The model under review builds one solid part; all positions refer to its coordinate system, in mm. A direction names the side the tool comes from. Coordinates: 2 decimals unless noted, no trailing zeros. Order: outer loops, then holes, each group sorted by start corner. A loop starts at its lowest first (then second) coordinate and runs counter-clockwise, first axis right, second up. Notation, with made-up numbers: M -33,4 L -6,4 A30 ccw -6,31 Z; hole C 45,22.5 d7. An arc over 180 degrees is marked long. Write each question's results on one line, items separated by ' | '.
from build123d import *

# Parameters (mm, degrees)
BOSS_EXTRUDE1_DEPTH     = 24
SKETCH2_W               = 3
SKETCH2_H               = 4
CUT_EXTRUDE1_DEPTH      = 4.1
BOSS_EXTRUDE2_DEPTH     = 0.8
SKETCH5_W               = 0.5
SKETCH5_H               = 0.5
CUT_EXTRUDE2_DEPTH      = 2
CUT_EXTRUDE2_DEPTH_BACK = 2
SKETCH6_W               = 1.8
SKETCH6_H               = 1.2
CUT_EXTRUDE3_DEPTH      = 0.1
SKETCH7_W               = 3
SKETCH7_H               = 1.3


with BuildPart() as part:
    # Sketch1 → Boss-Extrude1 (new body)
    with BuildSketch(Plane(origin=(0, 0, 0), x_dir=(0, 0, -1), z_dir=(1, 0, 0))):
        with BuildLine():
            Line((-2.7, 0.6), (-1.428285686, 0.6))
            ThreePointArc((-1.428285686, 0.6), (2, 2), (-1.428285686, 3.4))
            Line((-1.428285686, 3.4), (-2.7, 3.4))
            Line((-2.7, 3.4), (-2.7, 0.6))
        make_face()
    extrude(amount=BOSS_EXTRUDE1_DEPTH)

    # Sketch2 → Cut-Extrude1 (cut)
    with BuildSketch(Plane(origin=(0, 0, 0), x_dir=(0, 0, -1), z_dir=(1, 0, 0))):
        with Locations((-1.2, 2)):
            Rectangle(SKETCH2_W, SKETCH2_H)
    extrude(amount=CUT_EXTRUDE1_DEPTH, mode=Mode.SUBTRACT)

    # Sketch3 → Boss-Extrude2 (add)
    with BuildSketch(Plane.XY.offset(-0.3)):
        with BuildLine():
            Line((0.4, 0.1), (3.6, 0.1))
            ThreePointArc((3.6, 0.1), (3.812132034, 0.187867966), (3.9, 0.4))
            Line((3.9, 0.4), (3.9, 3.6))
            ThreePointArc((3.9, 3.6), (3.812132034, 3.812132034), (3.6, 3.9))
            Line((3.6, 3.9), (0.4, 3.9))
            ThreePointArc((0.4, 3.9), (0.187867966, 3.812132034), (0.1, 3.6))
            Line((0.1, 3.6), (0.1, 0.4))
            ThreePointArc((0.1, 0.4), (0.187867966, 0.187867966), (0.4, 0.1))
        make_face()
    extrude(amount=BOSS_EXTRUDE2_DEPTH)

    # Sketch4 → Revolve1 (revolve)
    with BuildSketch(Plane(origin=(0, 2, 0), x_dir=(-1, 0, 0), z_dir=(0, 1, 0))):
        Polygon((-2, 2.55), (-0.5, 2.55), (-0.5, 2.05), (0, 1.55), (0, 0.65), (-1.25, 0.65), (-1.25, 0.3), (-2, 0.3), align=None)
    revolve(axis=Axis((2, 2, 0.3), (0, 0, 1)))

    # Sketch5 → Cut-Extrude2 (cut, two sides)
    with BuildSketch(Plane(origin=(0, 2, 0), x_dir=(-1, 0, 0), z_dir=(0, 1, 0))) as cut_extrude2_sk:
        with Locations((-2, 2.3)):
            Rectangle(SKETCH5_W, SKETCH5_H)
    extrude(amount=CUT_EXTRUDE2_DEPTH, mode=Mode.SUBTRACT)
    extrude(cut_extrude2_sk.sketch, amount=-CUT_EXTRUDE2_DEPTH_BACK, mode=Mode.SUBTRACT)

    # Sketch6 → Cut-Extrude3 (cut)
    with BuildSketch(Plane.XY.offset(2.7)):
        with Locations((14.9, 2)):
            Rectangle(SKETCH6_W, SKETCH6_H)
    extrude(amount=-CUT_EXTRUDE3_DEPTH, mode=Mode.SUBTRACT)

    # Sketch7 → Revolve2 (revolve)
    with BuildSketch(Plane(origin=(0, 2, 0), x_dir=(-1, 0, 0), z_dir=(0, 1, 0))):
        with Locations((-25.5, -0.65)):
            Rectangle(SKETCH7_W, SKETCH7_H)
    revolve(axis=Axis((27, 2, 0), (-1, 0, 0)))


solid = part.part
1) For faces 4 (the flat face through (1, 2, 0.65)), 5 (the flat face through (4.1, 2, 2)), 6 (the cylindrical face through (0.5, 2, 2.3)), 7 (the flat face through (3, 2, 2.55)), 8 (the flat face through (15, 2, 2.6)), list the 3-axis set-ups (+Z, -Z, +X, -X, +Y, -Y) from which the entire face can be reached by the end or side of a thin tool; tool diameter is ignored.
Solutions:
face 4: none | face 5: +Z, +Y, -Y | face 6: +Z, -X | face 7: +Z, -X, +Y, -Y | face 8: +Z
2) Take a section at B-B on x = 2. State the section outline as (y, z) points, plus the area to 3 significant figures.
Solutions:
outline: M 0,0.65 L 1.25,0.65 L 1.25,0.5 L 0.1,0.5 L 0.1,-0.3 L 0.02,-0.3 A2 ccw 3.98,-0.3 L 3.9,-0.3 L 3.9,0.5 L 2.75,0.5 L 2.75,0.65 L 4,0.65 L 4,1.55 L 3.5,2.05 L 0.5,2.05 L 0,1.55 Z | area: 13.7 mm2
3) For pin 1 (1.4 mm diameter, centred on x = 12, z = 2, fed in from -Y); pin 2 (1.3 mm diameter, centred on x = 15, y = 2, fed in from +Z); pin 3 (1.5 mm diameter, centred on x = 8, y = 3, fed in from -Z); pin 4 (0.6 mm diameter, centred on x = 1, y = 1.5, fed in from +Z), all flat-tipped, find the tip position at first contact; note any pin that passes through.
Solutions:
pin 1: y = 0.48 | pin 2: z = 2.7 | pin 3: z = -1.98 | pin 4: z = 2.55
4) Take a section at A-A on z = 0. State the section outline as (x, y) points.
Solutions:
outline: M 0.1,0.4 A0.3 ccw 0.4,0.1 L 3.6,0.1 A0.3 ccw 3.9,0.4 L 3.9,3.6 A0.3 ccw 3.6,3.9 L 0.4,3.9 A0.3 ccw 0.1,3.6 Z; M 4.1,0 L 24,0 L 24,0.7 L 27,0.7 L 27,3.3 L 24,3.3 L 24,4 L 4.1,4 Z
5) The part is to be moulded in two halves that separate along Z. For faces 1 (the cylindrical face through (12, 2, -2)), 2 (the flat face through (3, 2, 0.5)), 3 (the flat face through (0, 2, -1)), say which applies: pulls with the +Z half, pulls with the -Z half, needs draft (parallel to the pull), parting line crosses it, or undercut.
Solutions:
face 1: parting line crosses it | face 2: undercut | face 3: needs draft
6) To check wall thickness, follow line 1 along X through (y, z) = (1.95, -0.05); line 2 along Y through (x, z) = (17.5, 1.75); line 3 along X through (y, z) = (0.75, -0.9). State the ranges of each line that lie inside material, in increasing order.
Solutions:
line 1: 0.1 to 3.9, 4.1 to 27 | line 2: 0.6 to 3.4 | line 3: 0 to 24
7) Take a section at D-D on x = 23.5. State the section outline as (y, z) points.
Solutions:
outline: M 0.6,1.43 A2 ccw long 3.4,1.43 L 3.4,2.7 L 0.6,2.7 Z
